```python
from build123d import *

# Parameters (mm, degrees)
BASIC_DEPTH             = 3.3
BEARING_START           = -2.1
SKETCH2_R               = 1.5
BEARING_CLEARANCE_DEPTH = 2.1
TOP_CLEARANCE_DEPTH     = 8.61905506
FILLET_R1_R             = 1
FILLET_R0_5_R           = 0.5
CHAMFER_R0_3_45_SIZE    = 0.3


with BuildPart() as part:
    # Sketch1 → Basic (new body)
    with BuildSketch(Plane.XY):
        with BuildLine():
            Line((4.2, -0.4), (4.2, -6))
            Line((4.2, -6), (-4.2, -6))
            Line((-4.2, -6), (-4.2, -0.4))
            ThreePointArc((-4.2, -0.4), (0, 3.8), (4.2, -0.4))
        make_face()
    extrude(amount=BASIC_DEPTH)

    # Sketch2 → Bearing Clearance (cut)
    with BuildSketch(Plane.XY.offset(3.3).offset(BEARING_START)):
        with BuildLine():
            Line((-4.2, -3), (-3.059411708, -3))
            ThreePointArc((-3.059411708, -3), (0, -4.2), (3.059411708, -3))
            Line((3.059411708, -3), (4.2, -3))
            Line((4.2, -3), (4.2, -0.4))
            ThreePointArc((4.2, -0.4), (0, 3.8), (-4.2, -0.4))
            Line((-4.2, -0.4), (-4.2, -3))
        make_face()
        with Locations((0, 0.3)):
            Circle(SKETCH2_R, mode=Mode.SUBTRACT)
    extrude(amount=BEARING_CLEARANCE_DEPTH, mode=Mode.SUBTRACT)

    # Sketch3 → Top Clearance (cut, through all)
    with BuildSketch(Plane.XY.offset(1.2)):
        with BuildLine():
            Line((-1.788854382, 3.4), (1.788854382, 3.4))
            ThreePointArc((1.788854382, 3.4), (0, 3.8), (-1.788854382, 3.4))
        make_face()
    extrude(amount=-TOP_CLEARANCE_DEPTH, mode=Mode.SUBTRACT)

    # Sketch7 → Bearing Get Low (revolve, cut)
    with BuildSketch(Plane(origin=(0, 0, 0), x_dir=(0, 0, -1), z_dir=(1, 0, 0)), mode=Mode.PRIVATE) as bearing_get_low_sk:
        with BuildLine():
            Line((-1.2, 1.8), (-1.2, 2.4))
            ThreePointArc((-1.2, 2.4), (-0.9, 2.1), (-1.2, 1.8))
        make_face()
    revolve(bearing_get_low_sk.sketch.rotate(Axis((0, 0.3, 3.3), (0, 0, -1)), 180), axis=Axis((0, 0.3, 3.3), (0, 0, -1)), mode=Mode.SUBTRACT)

    # R1
    fillet_r1_edges = [part.edges().sort_by_distance(p)[0] for p in [
        (-1.788854382, 3.4, 0.6),
        (1.788854382, 3.4, 0.6),
        (-4.2, -6, 1.65),
        (4.2, -6, 1.65),
    ]]
    fillet(fillet_r1_edges, radius=FILLET_R1_R)

    # R0.5
    fillet_r0_5_edges = [part.edges().sort_by_distance(p)[0] for p in [
        (-4.2, -3, 2.25),
        (-3.059411708, -3, 2.25),
        (3.059411708, -3, 2.25),
        (4.2, -3, 2.25),
    ]]
    fillet(fillet_r0_5_edges, radius=FILLET_R0_5_R)

    # R0.3×45°
    chamfer_r0_3_45_edges = [part.edges().sort_by_distance(p)[0] for p in [
        (-1.5, 0.3, 3.3),
    ]]
    chamfer(chamfer_r0_3_45_edges, length=CHAMFER_R0_3_45_SIZE)


solid = part.part
```
Input: part model. Units: mm. Frame: model coordinates. A direction names the side the tool comes from. Round coordinates to 2 decimals unless told otherwise and drop trailing zeros. Write each loop counter-clockwise with the first axis right and the second up, starting at its lowest first coordinate (ties: lowest second). Pieces come first, ordered by that corner, then holes. Notation, with made-up numbers: (-13.5, 24) - (11.5, 24) arc R29 cw to (11.5, 62) - close; hole circle Ø2 at (78, 12.5). An arc over 180 degrees is marked (long way). Write item = value, one per line.
(1) Pull-direction query (X, two-part tool) for faces 1 (the cylindrical face through (0, -4.2, 2.2)), 2 (the cylindrical face through (3.6, 1.76, 0.59)), 3 (the flat face through (0, 3.4, 1)); classes: +X half, -X half, draft (parallel to the pull), parting line (faces both ways), or undercut.
Geometry check:
face_1 = undercut
face_2 = +X half
face_3 = draft
(2) Access query for faces 4 (the cylindrical face through (-3.899, -5.715, 1.673)), 5 (the cylindrical face through (-1.5, 0.37, 2.09)). Directions: +Z, -Z, +X, -X, +Y, -Y. A direction counts if a zero-diameter tool reaches every point of the face in a straight line with its end or side. Return the directions, or none.
Geometry check:
face_4 = +Z, -Z, -X, -Y
face_5 = +Z
(3) Section query C-C on x = -2.75. Output: boundary loops of the cut face in (y, z).
Geometry check:
outline = (-6, 0) - (2.77, 0) - (2.77, 1.2) - (-3.26, 1.2) - (-3.26, 3.3) - (-6, 3.3) - close
(4) Contact query for a flat-ended pin moving along its axis: pin 1 Ø1 at (y, z) = (1.5, 1) entering from -X. Output: stop coordinate, or through.
Geometry check:
pin_1 = -3.96
(5) Section query B-B on y = 0.3. Output: boundary loops of the cut face in (x, z), then the cut area to 3 significant figures.
Geometry check:
outline = (-4.14, 0) - (4.14, 0) - (4.14, 1.2) - (2.1, 1.2) arc R0.3 cw to (1.5, 1.2) - (1.5, 3) - (1.2, 3.3) - (-1.2, 3.3) - (-1.5, 3) - (-1.5, 1.2) arc R0.3 cw to (-2.1, 1.2) - (-4.14, 1.2) - close
area = 15.9 mm^2
(6) Material intervals for probe 1 along X at (y, z) = (1, 1.05); probe 2 along Z at (x, y) = (1.25, 2.5); probe 3 along Y at (x, z) = (-0.75, 1.55), sorted ascending.
Geometry check:
probe_1 = -3.96 to -1.94, -1.37 to 1.37, 1.94 to 3.96
probe_2 = 0 to 1.2
probe_3 = -6 to -4.14, -1 to 1.6
(7) Section query A-A on x = 0. Output: boundary loops of the cut face in (y, z), then the cut area to 3 significant figures.
Geometry check:
outline = (-6, 0) - (3.4, 0) - (3.4, 1.2) - (2.4, 1.2) arc R0.3 cw to (1.8, 1.2) - (1.8, 3) - (1.5, 3.3) - (-0.9, 3.3) - (-1.2, 3) - (-1.2, 1.2) arc R0.3 cw to (-1.8, 1.2) - (-4.2, 1.2) - (-4.2, 3.3) - (-6, 3.3) - close
area = 21.0 mm^2
